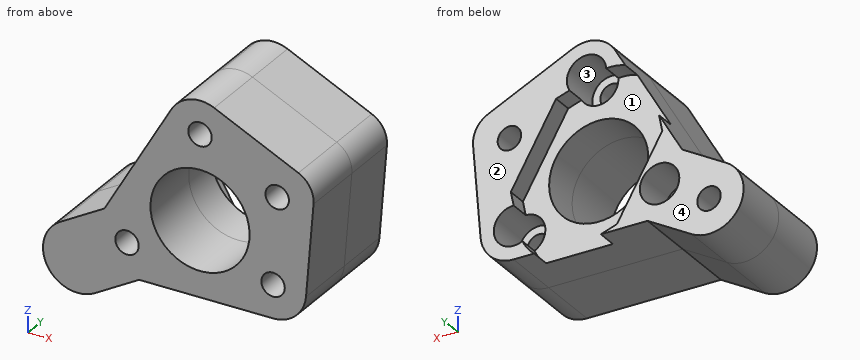
Solid Edge part; units mm, degrees
sketch "Sketch1" plane through (0, 0, 0) normal (0, -1, 0) x (1, 0, 0)
  line L0 (-5.3694, 18.9) -> (-19.0694, -4.8291)
  arc A0 (-13.7, -14.1291) -> (-19.0694, -4.8291) centre (-13.7, -7.9291) cw
  line L1 (-13.7, -14.1291) -> (13.7, -14.1291)
  arc A1 (19.0694, -4.8291) -> (13.7, -14.1291) centre (13.7, -7.9291) cw
  line L2 (5.3694, 18.9) -> (19.0694, -4.8291)
  arc A2 (-5.3694, 18.9) -> (5.3694, 18.9) centre (0, 15.8) cw
  dimension "D1" = 5.3694
extrude "Protrusion1" add sketch "Sketch1" against normal blind 14
sketch "Sketch2" plane through (0, 0, 0) normal (0, -1, 0) x (1, 0, 0)
  circle A0 centre (-13.7, -7.9291) radius 2.2
  circle A1 centre (13.7, -7.9291) radius 2.2
  circle A2 centre (0, 15.8) radius 2.2
extrude "Cutout1" cut sketch "Sketch2" against normal blind 457.8755
sketch "Sketch3" plane through (0, 0, 0) normal (0, -1, 0) x (1, 0, 0)
  circle A0 centre (0, 0) radius 9.3
extrude "Cutout2" cut sketch "Sketch3" against normal blind 434.4917
sketch "Sketch4" plane through (0, 0, 3.9355) normal (0, -1, 0) x (-0.5, 0, 0.8660254)
  line L0 (-23.325, -5.9323) -> (-23.325, -18.9323)
  line L1 (-23.325, -18.9323) -> (16.475, -18.9323)
  line L2 (16.475, -18.9323) -> (16.475, -5.9323)
  line L3 (12.7755, -8.7037) -> (16.475, -5.9323)
  line L4 (-20.9306, -8.7037) -> (12.7755, -8.7037)
  line L5 (-20.9306, -5.9323) -> (-20.9306, -8.7037)
  line L6 (-23.325, -5.9323) -> (-20.9306, -5.9323)
  dimension "D1" = 23.325
extrude "Protrusion2" add sketch "Sketch4" against normal up to vertex (14 mm away)
sketch "Sketch5" plane through (18.1083, 8, 10.4355) normal (0.8660254, 0, 0.5) x (-0.5, 0, 0.8660254)
  line L0 (-19.9, 8) -> (19.9, 8)
  line L1 (19.9, -6) -> (19.9, 8)
  line L2 (-19.9, -6) -> (19.9, -6)
  line L3 (-19.9, -6) -> (-19.9, 8)
extrude "ExtrudedProtrusion_14" add sketch "Sketch5" along normal blind 4
sketch "Sketch6" plane through (5.8112, 14, 7.7701) normal (0, 1, 0) x (0.5, 0, -0.8660254)
  circle A0 centre (3.8403, 24.7468) radius 3.7
  circle A1 centre (17.5403, 1.0177) radius 3.7
  circle A2 centre (-9.8597, 1.0177) radius 3.7
extrude "Cutout3" cut sketch "Sketch6" against normal blind 8
sketch "Sketch7" plane through (11.8615, 14, 7.7701) normal (0, 1, 0) x (-0.8660254, 0, -0.5)
  circle A0 centre (-2.5426, -0.8152) radius 2.2
extrude "ExtrudedCutout_23" cut sketch "Sketch7" against normal blind 166.5817
sketch "Sketch8" plane through (11.8615, 14, 7.7701) normal (0, 1, 0) x (-0.8660254, 0, -0.5)
  circle A0 centre (40.6865, -0.8152) radius 2.2
  line L0 (40.6865, 5.6848) -> (31.1282, 5.6848)
  line L1 (31.1282, 5.6848) -> (31.1282, 3.8832)
  line L2 (31.1282, 3.8832) -> (34.2429, 1.8592)
  line L3 (34.2429, 1.8592) -> (34.2429, -2.6486)
  line L4 (31.1282, -7.3152) -> (34.2429, -2.6486)
  line L5 (40.6865, -7.3152) -> (31.1282, -7.3152)
  arc A1 (40.6865, -7.3152) -> (40.6865, 5.6848) centre (40.6865, -0.8152) ccw
extrude "Protrusion3" add sketch "Sketch8" against normal up to vertex (14 mm away)
sketch "Sketch9" plane through (11.8615, 14, 7.7701) normal (0, 1, 0) x (-0.8660254, 0, -0.5)
  line L0 (-10.7426, -0.8152) -> (-10.7426, -20.7152)
  line L1 (-10.7426, -20.7152) -> (6.2574, -20.7152)
  arc A0 (1.1563, -18.0392) -> (6.2574, -20.7152) centre (6.2574, -14.5152) ccw
  line L2 (1.1563, -18.0392) -> (-10.7426, -0.8152)
extrude "Cutout4" cut sketch "Sketch9" against normal blind 85.4791
sketch "Sketch10" plane through (6.8865, 14, 7.7701) normal (0, 1, 0) x (-0.8660254, 0, -0.5)
  line L0 (-15.0511, 16.5973) -> (-15.0511, -3.3027)
  line L1 (-3.1522, 13.9213) -> (-15.0511, -3.3027)
  arc A0 (1.9489, 16.5973) -> (-3.1522, 13.9213) centre (1.9489, 10.3973) ccw
  line L2 (1.9489, 16.5973) -> (-15.0511, 16.5973)
extrude "ExtrudedCutout_27" cut sketch "Sketch10" against normal blind 118.3722
sketch "Sketch11" plane through (0, 0, 0) normal (0, 0, 1) x (1, 0, 0)
  line L0 (-57, 0) -> (32.4619, 0)
  line L1 (32.4619, 0) -> (32.4619, 3)
  line L2 (32.4619, 3) -> (-57, 3)
  line L3 (-57, 3) -> (-57, 0)
  dimension "D1" = 57
extrude "Cutout5" cut sketch "Sketch11" along normal mid plane 82.8276
sketch "Sketch12" plane through (11.8615, 14, 7.7701) normal (0, 1, 0) x (-0.8660254, 0, -0.5)
  line L0 (2.6574, 7.7016) -> (2.6574, -9.2984)
  line L1 (2.6574, -9.2984) -> (7.9574, -15.2984)
  arc A0 (20.3574, -15.2984) -> (7.9574, -15.2984) centre (14.1574, -9.8217) cw
  line L2 (25.6574, -9.2984) -> (20.3574, -15.2984)
  line L3 (25.6574, 7.7016) -> (25.6574, -9.2984)
  line L4 (25.6574, 7.7016) -> (20.3574, 13.7016)
  arc A1 (7.9574, 13.7016) -> (20.3574, 13.7016) centre (14.1574, 8.2249) cw
  line L5 (2.6574, 7.7016) -> (7.9574, 13.7016)
extrude "Cutout6" cut sketch "Sketch12" against normal blind 3.8
fillet "Round_2" radius 5 1 edges at (21.5724, 8.5, 12.4355)
sketch "Sketch13" plane through (-4.0785, 3, 1.1105) normal (0, -1, 0) x (-0.0808589, 0, -0.9967256)
  line L0 (-14.5843, 21.4205) -> (-20.7701, 5.0713)
  arc A0 (-17.6269, -2.7251) -> (-20.7701, 5.0713) centre (-14.9712, 2.8773) cw
  line L1 (-17.6269, -2.7251) -> (5.0889, -13.4929)
  line L2 (10.5218, -21.3571) -> (5.0889, -13.4929)
  arc A1 (21.2176, -13.9681) -> (10.5218, -21.3571) centre (15.8697, -17.6626) cw
  line L3 (15.7848, -6.1039) -> (21.2176, -13.9681)
  line L4 (13.7521, 18.9525) -> (15.7848, -6.1039)
  arc A2 (7.5724, 24.6512) -> (13.7521, 18.9525) centre (7.5724, 18.4512) cw
  line L5 (7.5724, 24.6512) -> (-9.9079, 24.6512)
  arc A3 (-14.5843, 21.4205) -> (-9.9079, 24.6512) centre (-9.9079, 19.6512) cw
  circle A4 centre (7.5724, 18.4512) radius 2.2
  circle A5 centre (-8.7012, 17.9046) radius 2.2
  circle A6 centre (-14.9712, 2.8773) radius 2.2
  circle A7 centre (0.777, 4.1549) radius 9.3
  circle A8 centre (9.7879, -8.8591) radius 2.2
extrude "ExtrudedProtrusion_16" add sketch "Sketch13" along normal blind 12
Build history of the part. All positions in model axes, mm. Face numbers are marked on the shaded views. A direction names the side the tool comes from. Give positions to 0.01 mm unless a question says otherwise; leave off trailing zeros. Order: outer loops, then holes, each group sorted by start corner. A loop starts at its lowest first (then second) coordinate and runs counter-clockwise, first axis right, second up. Notation, with made-up numbers: M -26.75,31 L 2.25,31 A29 ccw 2.25,52 Z; hole C 13.5,71 d6. An arc over 180 degrees is marked long. Use one line per item in the form item = value.
1) Drop flat-ended pins along their axis: pin 1 (2 mm diameter, centred on x = 1, z = 15.5, fed in from +Y); pin 2 (9 mm diameter, centred on x = -4, y = 9.5, fed in from -Z); pin 3 (8.5 mm diameter, centred on x = -4, z = 5, fed in from +Y); pin 4 (5 mm diameter, centred on x = 0, z = 15.8, fed in from +Y). Give the stop position or say it passes through.
Calculated:
pin_1 = through
pin_2 = -14.13
pin_3 = 10.2
pin_4 = 6
2) Two-plate mould, pull along Z, no slides. Class the marked faces 3 and 4: released by +Z, released by -Z, zero draft, split by the parting line, or undercut.
Calculated:
face_3 = undercut
face_4 = zero draft
3) Tool access for the marked faces 1 and 2: list every direction of +Z, -Z, +X, -X, +Y, -Y with a clear straight run to the whole face (end or side of a thin tool).
Calculated:
face_1 = +Y
face_2 = +Z, -Z, +X, -X, +Y
4) Probe probe 1 along Z at (x, y) = (0, 7); probe 2 along X at (y, z) = (0, 7); probe 3 along Z at (x, y) = (15, -6.25). List the from-to ranges inside material, lowest first.
Calculated:
probe_1 = -14.13 to -9.3, 9.3 to 12.1, 19.5 to 22
probe_2 = -12.24 to -6.12, 6.12 to 12.72, 16.22 to 21.13
probe_3 = -13.99 to -9.7, -6.15 to 6.2, 10.47 to 15.55
5) Saw through at C-C (y = -2.75). Give the cut face in (x, z).
Calculated:
outline = M -26.22,-7.65 A6.5 ccw -19.72,-18.91 L -11.44,-14.13 L 13.7,-14.13 A6.2 ccw 19.88,-8.43 L 21.29,8.99 A5 ccw 18.45,13.92 L 2.66,21.4 A6.2 ccw -5.37,18.9 L -17.94,-2.87 Z; hole C -13.7,-7.93 d4.4; hole C 0,0 d18.6; hole C 0,15.8 d4.4; hole C 13.7,-7.93 d4.4; hole C 14.47,8.34 d4.4
6) Saw through at B-B (x = -1.5). Give the cut face in (y, z), plus the area to 3 significant figures.
Calculated:
outline = M -9,-14.13 L 10.2,-14.13 L 10.2,-9.18 L -9,-9.18 Z; M -9,9.18 L 10.2,9.18 L 10.2,12.42 L 6,12.42 L 6,14.19 L -9,14.19 Z; M -9,17.41 L 6,17.41 L 6,19.18 L 14,19.18 L 14,21.82 L -9,21.82 Z
area = 271 mm2
7) Saw through at A-A (x = 5). Give the cut face in (y, z), plus the area to 3 significant figures.
Calculated:
outline = M -9,-14.13 L 10.2,-14.13 L 10.2,-7.84 L -9,-7.84 Z; M -9,7.84 L 10.2,7.84 L 10.2,13.35 L 14,13.35 L 14,20.29 L -9,20.29 Z
area = 386 mm2
